Input: part model. Units: mm. Frame: model coordinates. Face numbers are marked on the shaded views. A direction names the side the tool comes from. Coordinates: 2 decimals unless noted, no trailing zeros. Order: outer loops, then holes, each group sorted by start corner. A loop starts at its lowest first (then second) coordinate and runs counter-clockwise, first axis right, second up. Notation, with made-up numbers: M 31,50 L 63,50 A17 cw 63,73 Z; hole C -16,36 d1. An arc over 180 degrees is marked long. One line per item, written item: value.
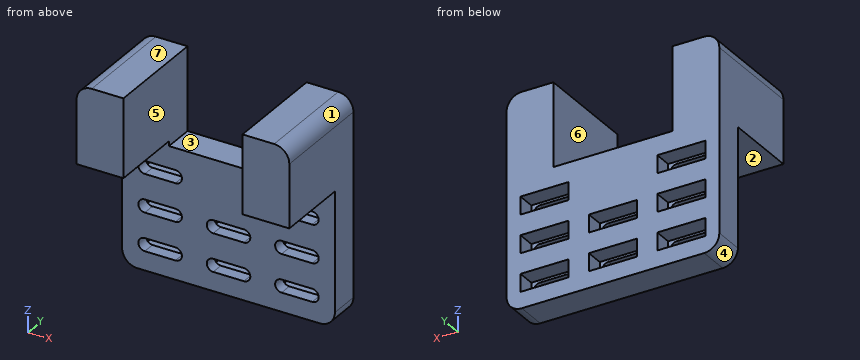
```python
from build123d import *

# Parameters (mm, degrees)
SKETCH1_W            = 44
SKETCH1_H            = 44
BOSS_EXTRUDE1_DEPTH  = 6
CUT_EXTRUDE1_DEPTH   = 7
SKETCH4_W            = 44
SKETCH4_H            = 16.5
BOSS_EXTRUDE2_DEPTH  = 14.75
SKETCH5_W            = 23.5
SKETCH5_H            = 17.45
CUT_EXTRUDE2_DEPTH   = 21.75
FILLET1_R            = 3
SKETCH6_W            = 9.5
SKETCH6_H            = 3.5
CUT_EXTRUDE3_DEPTH   = 3.52
LPATTERN1_COUNT      = 3
LPATTERN1_PITCH      = 13.5
LPATTERN1_COUNT_DIR2 = 3
LPATTERN1_PITCH_DIR2 = 7.5
CUT_EXTRUDE5_REACH   = 22.75


with BuildPart() as part:
    # Sketch1 → Boss-Extrude1 (new body)
    with BuildSketch(Plane(origin=(0, 0, 0), x_dir=(1, 0, 0), z_dir=(0, 1, 0))):
        with Locations((22, 22)):
            Rectangle(SKETCH1_W, SKETCH1_H)
    extrude(amount=-BOSS_EXTRUDE1_DEPTH)

    # Sketch2 → Cut-Extrude1 (cut, through all)
    with BuildSketch(Plane(origin=(0, 0, 0), x_dir=(1, 0, 0), z_dir=(0, 1, 0))):
        with BuildLine():
            Line((5.475, 39.275), (11.525, 39.275))
            ThreePointArc((11.525, 39.275), (12.8, 38), (11.525, 36.725))
            Line((11.525, 36.725), (5.475, 36.725))
            ThreePointArc((5.475, 36.725), (4.2, 38), (5.475, 39.275))
        make_face()
        with BuildLine():
            Line((18.975, 39.275), (25.025, 39.275))
            ThreePointArc((25.025, 39.275), (26.3, 38), (25.025, 36.725))
            Line((25.025, 36.725), (18.975, 36.725))
            ThreePointArc((18.975, 36.725), (17.7, 38), (18.975, 39.275))
        make_face()
        with BuildLine():
            Line((32.475, 39.275), (38.525, 39.275))
            ThreePointArc((38.525, 39.275), (39.8, 38), (38.525, 36.725))
            Line((38.525, 36.725), (32.475, 36.725))
            ThreePointArc((32.475, 36.725), (31.2, 38), (32.475, 39.275))
        make_face()
        with BuildLine():
            Line((18.975, 31.775), (25.025, 31.775))
            ThreePointArc((25.025, 31.775), (26.3, 30.5), (25.025, 29.225))
            Line((25.025, 29.225), (18.975, 29.225))
            ThreePointArc((18.975, 29.225), (17.7, 30.5), (18.975, 31.775))
        make_face()
        with BuildLine():
            Line((32.475, 31.775), (38.525, 31.775))
            ThreePointArc((38.525, 31.775), (39.8, 30.5), (38.525, 29.225))
            Line((38.525, 29.225), (32.475, 29.225))
            ThreePointArc((32.475, 29.225), (31.2, 30.5), (32.475, 31.775))
        make_face()
        with BuildLine():
            Line((32.475, 24.275), (38.525, 24.275))
            ThreePointArc((38.525, 24.275), (39.8, 23), (38.525, 21.725))
            Line((38.525, 21.725), (32.475, 21.725))
            ThreePointArc((32.475, 21.725), (31.2, 23), (32.475, 24.275))
        make_face()
        with BuildLine():
            Line((5.475, 31.775), (11.525, 31.775))
            ThreePointArc((11.525, 31.775), (12.8, 30.5), (11.525, 29.225))
            Line((11.525, 29.225), (5.475, 29.225))
            ThreePointArc((5.475, 29.225), (4.2, 30.5), (5.475, 31.775))
        make_face()
        with BuildLine():
            Line((5.475, 24.275), (11.525, 24.275))
            ThreePointArc((11.525, 24.275), (12.8, 23), (11.525, 21.725))
            Line((11.525, 21.725), (5.475, 21.725))
            ThreePointArc((5.475, 21.725), (4.2, 23), (5.475, 24.275))
        make_face()
    extrude(amount=-CUT_EXTRUDE1_DEPTH, mode=Mode.SUBTRACT)

    # Sketch4 → Boss-Extrude2 (add)
    with BuildSketch(Plane.XZ.offset(6)):
        with Locations((22, -8.25)):
            Rectangle(SKETCH4_W, SKETCH4_H)
    extrude(amount=BOSS_EXTRUDE2_DEPTH)

    # Sketch5 → Cut-Extrude2 (cut, through all)
    with BuildSketch(Plane(origin=(0, 0, 0), x_dir=(1, 0, 0), z_dir=(0, 1, 0))):
        with Locations((22, 8.725)):
            Rectangle(SKETCH5_W, SKETCH5_H)
    extrude(amount=-CUT_EXTRUDE2_DEPTH, mode=Mode.SUBTRACT)

    # Fillet1
    fillet1_edges = [part.edges().sort_by_distance(p)[0] for p in [
        (0, -10.375, 0),
        (44, -10.375, 0),
        (44, -3, -44),
        (0, -3, -44),
    ]]
    fillet(fillet1_edges, radius=FILLET1_R)

    # Sketch6 → Cut-Extrude3 (cut)
    with BuildSketch(Plane(origin=(0, 0, 0), x_dir=(1, 0, 0), z_dir=(0, 1, 0))):
        with Locations((8.5, 38)):
            Rectangle(SKETCH6_W, SKETCH6_H)
    cut_extrude3 = extrude(amount=-CUT_EXTRUDE3_DEPTH, mode=Mode.SUBTRACT)

    # LPattern1: Cut-Extrude3 3 × 3, 1 skipped
    with Locations(*[(i * LPATTERN1_PITCH, 0, j * LPATTERN1_PITCH_DIR2) for i in range(LPATTERN1_COUNT) for j in range(LPATTERN1_COUNT_DIR2) if (i, j) not in ((0, 0), (1, 2))]):
        add(cut_extrude3, mode=Mode.SUBTRACT)

    # Sketch7 → Cut-Extrude5 (cut, up to next)
    with BuildSketch(Plane(origin=(0, 0, 0), x_dir=(1, 0, 0), z_dir=(0, 1, 0)), mode=Mode.PRIVATE) as cut_extrude5_sk1:
        with BuildLine():
            Line((10.25, 0), (10.25, 1))
            Line((10.25, 1), (4, 1))
            ThreePointArc((4, 1), (1.878679656, 1.878679656), (1, 4))
            Line((1, 4), (1, 40))
            ThreePointArc((1, 40), (1.878679656, 42.121320344), (4, 43))
            Line((4, 43), (40, 43))
            ThreePointArc((40, 43), (42.121320344, 42.121320344), (43, 40))
            Line((43, 40), (43, 4))
            ThreePointArc((43, 4), (42.121320344, 1.878679656), (40, 1))
            Line((40, 1), (33.75, 1))
            Line((33.75, 1), (33.75, 0))
            Line((33.75, 0), (41, 0))
            ThreePointArc((41, 0), (43.121320344, 0.878679656), (44, 3))
            Line((44, 3), (44, 41))
            ThreePointArc((44, 41), (43.121320344, 43.121320344), (41, 44))
            Line((41, 44), (3, 44))
            ThreePointArc((3, 44), (0.878679656, 43.121320344), (0, 41))
            Line((0, 41), (0, 3))
            ThreePointArc((0, 3), (0.878679656, 0.878679656), (3, 0))
            Line((3, 0), (10.25, 0))
        make_face()
    cut_extrude5_tool1 = extrude(cut_extrude5_sk1.sketch, amount=-CUT_EXTRUDE5_REACH, mode=Mode.PRIVATE) & part.part
    add(cut_extrude5_tool1.solids().sort_by_distance((6.625, 0, -0.622254))[0], mode=Mode.SUBTRACT)


solid = part.part
```
(1) Cut plane C-C on z = -23. Output: boundary loops of the cut face in (x, y), plus the area to 3 significant figures.
Data:
outline: M 1,-6 L 4.2,-6 L 4.2,-3.52 L 3.75,-3.52 L 3.75,0 L 1,0 Z; M 12.8,-6 L 31.2,-6 L 31.2,-3.52 L 30.75,-3.52 L 30.75,0 L 13.25,0 L 13.25,-3.52 L 12.8,-3.52 Z; M 39.8,-6 L 43,-6 L 43,0 L 40.25,0 L 40.25,-3.52 L 39.8,-3.52 Z
area: 142 mm2
(2) First-contact query: pin 1 (1 mm diameter, centred on x = 6.5, z = -30.5, fed in from +Y); pin 2 (6 mm diameter, centred on x = 11.5, y = -13, fed in from -Z); pin 3 (10 mm diameter, centred on x = 8, y = -10.5, fed in from -Z); pin 4 (2.5 mm diameter, centred on x = 23, y = -5, fed in from +Z). Flat tips, straight axial feed; report the tip coordinate or a pass-through.
Data:
pin 1: passes through
pin 2: stops at z = -16.5
pin 3: stops at z = -43
pin 4: stops at z = -17.45
(3) Cut plane B-B on x = 22.5. Output: boundary loops of the cut face in (y, z) (3 decimals), plus the area to 3 significant figures.
Data:
outline: M -6,-43 L 0,-43 L 0,-39.75 L -3.52,-39.75 L -3.52,-39.275 L -6,-39.275 Z; M -6,-36.725 L -3.52,-36.725 L -3.52,-36.25 L 0,-36.25 L 0,-32.25 L -3.52,-32.25 L -3.52,-31.775 L -6,-31.775 Z; M -6,-29.225 L -3.52,-29.225 L -3.52,-28.75 L 0,-28.75 L 0,-17.45 L -6,-17.45 Z
area: 116 mm2
(4) Access query for the marked faces 1, 2 and 3. Directions: +Z, -Z, +X, -X, +Y, -Y. A direction counts if a zero-diameter tool reaches every point of the face in a straight line with its end or side. Return the directions, or none.
Data:
face 1: +Z, +X, +Y, -Y
face 2: -Z, +X, -X, -Y
face 3: +Z, +Y, -Y
(5) Draft query along X for the marked faces 4, 5, 6 and 7. Return one class per face: released by +X, released by -X, zero draft, split by the parting line, or undercut.
Data:
face 4: released by -X
face 5: undercut
face 6: undercut
face 7: zero draft
(6) Cut plane A-A on y = -9.5. Output: boundary loops of the cut face in (x, z).
Data:
outline: M 1,-16.5 L 10.25,-16.5 L 10.25,-1 L 4,-1 A3 ccw 1,-4 Z; M 33.75,-16.5 L 43,-16.5 L 43,-4 A3 ccw 40,-1 L 33.75,-1 Z
(7) Ray query, line 1 (Z direction, x = 8, y = -1.5); line 2 (X direction, y = -1.75, z = -23); line 3 (X direction, y = -14.75, z = -10). Return the intervals inside material, ascending. Write a range as from..to.
Data:
line 1: z = -43..-39.75, -36.25..-32.25, -28.75..-24.75, -21.25..-1
line 2: x = 1..3.75, 13.25..30.75, 40.25..43
line 3: x = 1..10.25, 33.75..43
(8) Cut plane D-D on z = -30.5. Output: boundary loops of the cut face in (x, y), plus the area to 3 significant figures.
Data:
outline: M 1,-6 L 4.2,-6 L 4.2,-3.52 L 3.75,-3.52 L 3.75,0 L 1,0 Z; M 12.8,-6 L 17.7,-6 L 17.7,-3.52 L 17.25,-3.52 L 17.25,0 L 13.25,0 L 13.25,-3.52 L 12.8,-3.52 Z; M 26.3,-6 L 31.2,-6 L 31.2,-3.52 L 30.75,-3.52 L 30.75,0 L 26.75,0 L 26.75,-3.52 L 26.3,-3.52 Z; M 39.8,-6 L 43,-6 L 43,0 L 40.25,0 L 40.25,-3.52 L 39.8,-3.52 Z
area: 87.7 mm2
